from build123d import *

# Parameters (mm, degrees)
BOSS_EXTRUDE2_DEPTH = 4
SKETCH2_R           = 0.5
SKETCH2_R_2         = 1.33
BOSS_EXTRUDE5_DEPTH = 3


with BuildPart() as part:
    # Sketch1 → Boss-Extrude2 (new body)
    with BuildSketch(Plane(origin=(0, 0, 0), x_dir=(1, 0, 0), z_dir=(0, 1, 0))):
        with BuildLine():
            ThreePointArc((27.5, -2.917608197), (29.999711791, -0.455568202), (27.575911257, 2.081239034))
            Line((27.575911257, 2.081239034), (0.857295011, 5.938437948))
            ThreePointArc((0.857295011, 5.938437948), (0.090022516, 5.999324624), (-0.678731386, 5.961486703))
            Line((-0.678731386, 5.961486703), (-27.424088743, 2.916455427))
            ThreePointArc((-27.424088743, 2.916455427), (-29.999711791, 0.455568202), (-27.5, -2.082391803))
            Line((-27.5, -2.082391803), (-0.859435998, -5.938128473))
            ThreePointArc((-0.859435998, -5.938128473), (-0.092185505, -5.999291778), (0.676581989, -5.961731025))
            Line((0.676581989, -5.961731025), (27.5, -2.917608197))
        make_face()
        with BuildLine():
            ThreePointArc((-17, -1.741842206), (-19, 0.258157794), (-17, 2.258157794))
            Line((-17, 2.258157794), (-0.65313587, 3.692683785))
            ThreePointArc((-0.65313587, 3.692683785), (-0.327822976, 3.735643465), (0, 3.75))
            ThreePointArc((0, 3.75), (0.43991732, 3.724106974), (0.873759552, 3.646785467))
            Line((0.873759552, 3.646785467), (17, 1.741842206))
            ThreePointArc((17, 1.741842206), (19, -0.258157794), (17, -2.258157794))
            Line((17, -2.258157794), (0.65313587, -3.692683785))
            ThreePointArc((0.65313587, -3.692683785), (0.327822976, -3.735643465), (0, -3.75))
            ThreePointArc((0, -3.75), (-0.43991732, -3.724106974), (-0.873759552, -3.646785467))
            Line((-0.873759552, -3.646785467), (-17, -1.741842206))
        make_face(mode=Mode.SUBTRACT)
    extrude(amount=BOSS_EXTRUDE2_DEPTH)

    # Sketch2 → Boss-Extrude5 (add)
    with BuildSketch(Plane(origin=(0, 4, 0), x_dir=(1, 0, 0), z_dir=(0, 1, 0))):
        with BuildLine():
            Line((27.580974078, 2.053213999), (0.863235763, 5.937577285))
            ThreePointArc((0.863235763, 5.937577285), (0.096028041, 5.999231502), (-0.6727599, 5.962163543))
            Line((-0.6727599, 5.962163543), (-27.419025922, 2.944162592))
            ThreePointArc((-27.419025922, 2.944162592), (-29.999672052, 0.485966647), (-27.5, -2.054525704))
            Line((-27.5, -2.054525704), (-0.865519194, -5.93724486))
            ThreePointArc((-0.865519194, -5.93724486), (-0.09833524, -5.999194128), (0.6704669, -5.962421835))
            Line((0.6704669, -5.962421835), (27.5, -2.945474296))
            ThreePointArc((27.5, -2.945474296), (29.999672052, -0.485966647), (27.580974078, 2.053213999))
        make_face()
        with Locations(Location((0, 0, 0), (0, 0, 270))):
            Circle(SKETCH2_R, mode=Mode.SUBTRACT)
        with Locations(Location((-14.45, 0.234076494, 0), (0, 0, 270))):
            Circle(SKETCH2_R_2, mode=Mode.SUBTRACT)
        with Locations(Location((14.45, -0.234076494, 0), (0, 0, 270))):
            Circle(SKETCH2_R_2, mode=Mode.SUBTRACT)
    extrude(amount=BOSS_EXTRUDE5_DEPTH)


solid = part.part
Geometry: final body of the model. Coordinates: model frame, mm. A direction names the side the tool comes from. Give positions to 0.01 mm unless a question says otherwise; leave off trailing zeros. Order: outer loops, then holes, each group sorted by start corner. A loop starts at its lowest first (then second) coordinate and runs counter-clockwise, first axis right, second up. Notation, with made-up numbers: (20.25, 34) -> (72.25, 34) arc R21 cw to (72.25, 66) -> close; hole circle Ø3 at (73, 7). An arc over 180 degrees is marked (long way). Answer as a JSON object with one key per item and string values.
Q1. Draft query along Z for faces 3 (the cylindrical face through (-0.488, 5.479, -0.108)), 4 (the cylindrical face through (30, 2, 0.5)), 5 (the flat face through (13.9, 1.97, 4.46)). Return one class per face: released by +Z, released by -Z, zero draft, split by the parting line, or undercut.
Entries:
{"face 3": "undercut", "face 4": "split by the parting line", "face 5": "released by +Z"}
Q2. Material intervals for probe 1 along X at (y, z) = (5.95, 0); probe 2 along X at (y, z) = (0.5, -1.5); probe 3 along X at (y, z) = (1, 1), sorted ascending.
Entries:
{"probe 1": "x = -29.96 to -15.76, -13.14 to -0.5, 0.5 to 13.14, 15.76 to 29.96", "probe 2": "x = -29.75 to -18.57, 17.95 to 29.1", "probe 3": "x = -29.56 to -18.55, 18.86 to 29.93"}
Q3. Access query for faces 1 (the flat face through (-14.366, 1.972, 3.983)), 2 (the flat face through (-8.941, 1.972, -2.965)). Directions: +Z, -Z, +X, -X, +Y, -Y. A direction counts if a zero-diameter tool reaches every point of the face in a straight line with its end or side. Return the directions, or none.
Entries:
{"face 1": "+Z, -X, +Y, -Y", "face 2": "-Y"}
Q4. First-contact query: pin 1 (3 mm diameter, centred on x = -2.5, y = 6, fed in from -Z); pin 2 (1.5 mm diameter, centred on x = 14.5, y = 5.5, fed in from -Z); pin 3 (4.5 mm diameter, centred on x = 20.5, z = 4, fed in from -Y); pin 4 (1.5 mm diameter, centred on x = -15, y = 1.5, fed in from +Z). Flat tips, straight axial feed; report the tip coordinate or a pass-through.
Entries:
{"pin 1": "stops at z = -5.93", "pin 2": "stops at z = -4.06", "pin 3": "stops at y = 0", "pin 4": "stops at z = 4"}
Q5. Section A-A (y = 4.5). Output: boundary loops of the cut face in (x, z).
Entries:
{"outline": "(-27.5, 2.05) arc R2.5 ccw (long way) to (-27.42, -2.94) -> (-0.67, -5.96) arc R6 ccw to (0.86, -5.94) -> (27.58, -2.05) arc R2.5 ccw to (27.5, 2.95) -> (0.67, 5.96) arc R6 ccw to (-0.87, 5.94) -> close; hole circle Ø2.66 at (-14.45, -0.23); hole circle Ø1 at (0, 0); hole circle Ø2.66 at (14.45, 0.23)"}
Q6. Section B-B (y = 1). Output: boundary loops of the cut face in (x, z), plus the area to 3 significant figures.
Entries:
{"outline": "(-27.5, 2.08) arc R2.5 ccw (long way) to (-27.42, -2.92) -> (-0.68, -5.96) arc R6 ccw to (0.86, -5.94) -> (27.58, -2.08) arc R2.5 ccw to (27.5, 2.92) -> (0.68, 5.96) arc R6 ccw to (-0.86, 5.94) -> close; hole (-17, -2.26) -> (-0.65, -3.69) arc R3.75 ccw to (0.87, -3.65) -> (17, -1.74) arc R2 ccw to (17, 2.26) -> (0.65, 3.69) arc R3.75 ccw to (-0.87, 3.65) -> (-17, 1.74) arc R2 ccw to start", "area": "282 mm^2"}
